```python
from build123d import *

# Parameters (mm, degrees)
F1_DEPTH = 19.05
F2_R     = 762
F3_R     = 38.1
F4_R     = 12.7


with BuildPart() as f1:
    # F0 (on Front) → F1 (new body)
    with BuildSketch(Plane.XZ):
        Polygon((157.48, 127), (0, 0), (914.4, 0), (607.290909, 101.6), (355.6, 304.8), (254, 304.8), align=None)
    extrude(amount=F1_DEPTH)

    # F2
    f2_edges = [f1.edges().sort_by_distance(p)[0] for p in [
        (157.48, -9.525, 127),
        (607.290909, -9.525, 101.6),
    ]]
    fillet(f2_edges, radius=F2_R)

    # F3
    f3_edges = [f1.edges().sort_by_distance(p)[0] for p in [
        (254, -9.525, 304.8),
        (355.6, -9.525, 304.8),
    ]]
    fillet(f3_edges, radius=F3_R)

    # F4
    f4_edges = [f1.edges().sort_by_distance(p)[0] for p in [
        (914.4, -9.525, 0),
        (0, -9.525, 0),
    ]]
    fillet(f4_edges, radius=F4_R)


solid = f1.part
```
Design review of the part built by this model. Coordinates are the model's own, in mm. Coordinates: 2 decimals unless noted, no trailing zeros. Order: outer loops, then holes, each group sorted by start corner. A loop starts at its lowest first (then second) coordinate and runs counter-clockwise, first axis right, second up. Notation, with made-up numbers: (-19.75, 3) - (-11.75, 3) arc R12 cw to (-11.75, 18) - close; hole circle Ø4 at (-7.75, -2.5). An arc over 180 degrees is marked (long way). One line per question, with ' | ' between items.
Q1. Consider section C-C, the plane x = 776.5. Give the boundary of the cut face in (y, z), then the cut area to 3 significant figures.
Answer key:
outline: (-19.05, 0) - (0, 0) - (0, 45.62) - (-19.05, 45.62) - close | area: 869 mm2
Q2. Consider section A-A, the plane y = -12.25. Give the boundary of the cut face in (x, z), then the cut area to 3 significant figures.
Answer key:
outline: (28.01, 22.59) arc R12.7 ccw to (35.98, 0) - (835.58, 0) arc R12.7 ccw to (839.57, 24.76) - (738.83, 58.08) arc R762 cw to (499.49, 188.63) - (366.07, 296.34) arc R38.1 ccw to (342.14, 304.8) - (276.67, 304.8) arc R38.1 ccw to (243.18, 284.88) - (230.19, 260.94) arc R762 cw to (38.85, 31.33) - close | area: 130,000 mm2
Q3. Clearance check with flat-ended pins moving along their axes: pin 1 Ø10 at (x, z) = (216, 154) entering from +Y; pin 2 Ø6 at (y, z) = (-10, 257) entering from -X. State where each tip first meets the part, or that it passes through.
Answer key:
pin 1: stops at y = 0 | pin 2: stops at x = 226.38
Q4. To check wall thickness, follow line 1 along X through (y, z) = (-17.25, 223); line 2 along X through (y, z) = (-7.25, 225.5); line 3 along Z through (x, y) = (802.5, -7.25). State the ranges of each line that lie inside material, in increasing order.
Answer key:
line 1: x = 208.16 to 456.92 | line 2: x = 209.7 to 453.82 | line 3: z = 0 to 37.02
Q5. Consider section B-B, the plane z = 216. Give the boundary of the cut face in (x, y), then the cut area to 3 significant figures.
Answer key:
outline: (203.77, -19.05) - (465.59, -19.05) - (465.59, 0) - (203.77, 0) - close | area: 4,990 mm2
